Check sheet for the drawn part. Datum: minimum x, y, z corner. Units: mm. Give positions to 0.01 mm unless a question says otherwise; leave off trailing zeros. Order: outer loops, then holes, each group sorted by start corner. A loop starts at its lowest first (then second) coordinate and runs counter-clockwise, first axis right, second up.
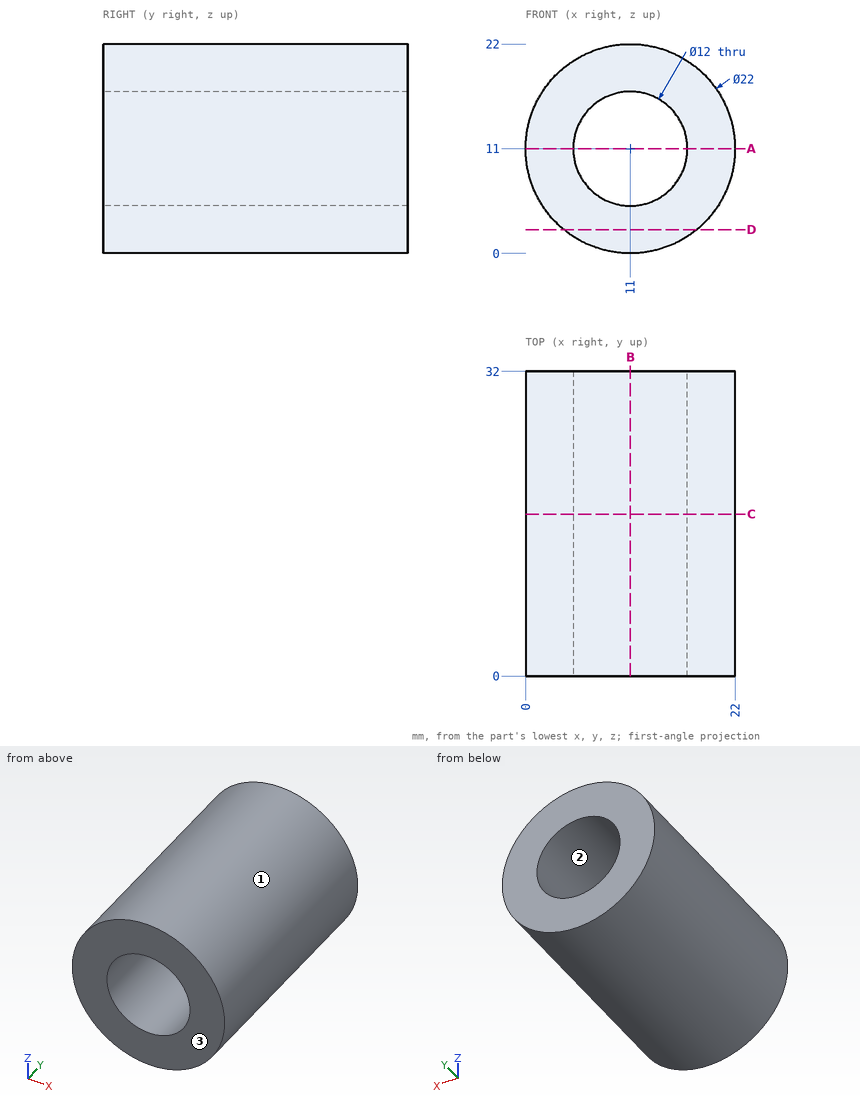
Q1. Go/stop test with flat-tipped pins: P1, Ø10, axis at y = 17.5, z = 3.5, coming from the -X side; P2, Ø8, axis at y = 15.5, z = 6.5, coming from the +X side; P3, Ø4, axis at y = 23.5, z = 19.5, coming from the -X side. Record where each tip stops, or that it passes through.
Q2. Draft check along Z on the marked faces 1, 2 and 3. Enter one of: pulls with the +Z half, pulls with the -Z half, needs draft (parallel to the pull), parting line crosses it, or undercut.
Q3. Sectioned sample at D-D, the plane z = 2.5. Record the cut outline in (x, y).
Q4. Sectioned sample at B-B, the plane x = 11. Record the cut outline in (y, z).
Q5. Sectioned sample at A-A, the plane z = 11. Record the cut outline in (x, y), plus the area to 3 significant figures.
Q6. Sectioned sample at C-C, the plane y = 17. Record the cut outline in (x, z), plus the area to 3 significant figures.
Q7. Material ranges on line 1 (X direction, y = 13, z = 10.75); line 2 (Z direction, x = 11, y = 12); line 3 (X direction, y = 30, z = 6.25), recorded low to high.
Filled in:
1. P1: stops at x = 0.29
1. P2: stops at x = 21.99
1. P3: stops at x = 2.13
2. face 1: parting line crosses it
2. face 2: undercut
2. face 3: needs draft
3. outline: (4.02, 0) - (17.98, 0) - (17.98, 32) - (4.02, 32) - close
4. outline: (0, 0) - (32, 0) - (32, 5) - (0, 5) - close; (0, 17) - (32, 17) - (32, 22) - (0, 22) - close
5. outline: (0, 0) - (5, 0) - (5, 32) - (0, 32) - close; (17, 0) - (22, 0) - (22, 32) - (17, 32) - close
5. area: 320 mm2
6. outline: circle Ø22 at (11, 11); hole circle Ø12 at (11, 11)
6. area: 267 mm2
7. line 1: x = 0 to 5.01, 16.99 to 22
7. line 2: z = 0 to 5, 17 to 22
7. line 3: x = 1.08 to 7.33, 14.67 to 20.92
